Build history of the part. All positions in model axes, mm. Face numbers are marked on the shaded views. A direction names the side the tool comes from. Round coordinates to 2 decimals unless told otherwise and drop trailing zeros. Loops run counter-clockwise (first coordinate to the right, second up) from the corner with the lowest first, then second, coordinate; pieces in that order, holes last. Notation, with made-up numbers: (32.25, 54) - (80.25, 54) arc R27 cw to (80.25, 87) - close; hole circle Ø6 at (-25.5, 69). An arc over 180 degrees is marked (long way). Put each result on its own line as item: value. Start each with the question number.
from build123d import *

# Parameters (mm, degrees)
F1_DEPTH = 50
F2_T     = -4
F3_R     = 15
F3_R_2   = 20
F4_DEPTH = 50.001
F5_R     = 5


with BuildPart() as f1:
    # F0 (on Front) → F1 (new body)
    with BuildSketch(Plane.XZ):
        Polygon((-95, -50), (95, -50), (95, 0), (53.363256, 50), (-95, 50), align=None)
    extrude(amount=-F1_DEPTH)

    # F2
    f2_openings = [f1.faces().sort_by_distance(p)[0] for p in [
        (-95, 25, 0),
        (95, 25, -25),
        (74.181628, 25, 25),
    ]]
    offset(amount=F2_T, openings=f2_openings)

    # F3 (on Front) → F4 (cut, through all)
    with BuildSketch(Plane.XZ):
        with Locations((-70, 25)):
            Circle(F3_R)
        with Locations((65, -20)):
            Circle(F3_R_2)
    extrude(amount=-F4_DEPTH, mode=Mode.SUBTRACT)

    # F5
    f5_edges = [f1.edges().sort_by_distance(p)[0] for p in [
        (-20.818372, 0, 50),
        (-20.818372, 50, 50),
        (0, 0, -50),
        (0, 50, -50),
    ]]
    fillet(f5_edges, radius=F5_R)


solid = f1.part
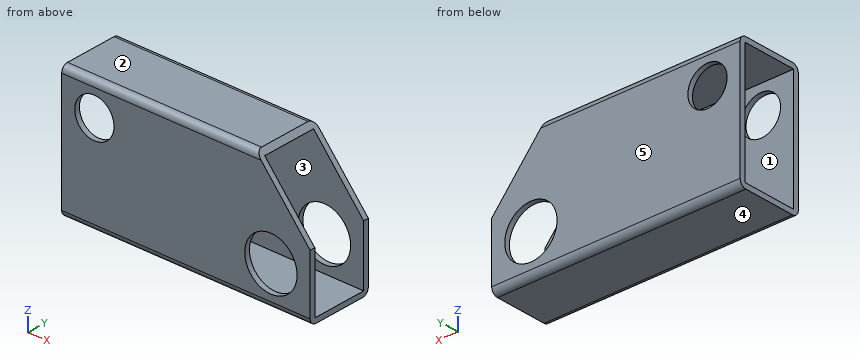
Item 1: Slice it at A-A (y = 8). Give the cut face in (x, z).
Item 2: Slice it at D-D (x = -70). Give the cut face in (y, z).
Item 3: Slice it at B-B (z = -20). Give the cut face in (x, y).
Item 4: Slice it at C-C (x = 27.5). Give the cut face in (y, z).
Item 5: Drill centre lines: probe 1 along Z at (x, y) = (-35, 32.5); probe 2 along Y at (x, z) = (66, 32); probe 3 along Z at (x, y) = (65, 49.15). Where is each one in solid material? Low to high. Write a range as [from, to].
Item 6: Two-plate mould, pull along Z, no slides. Class the marked faces 3, 4 and 5: pulls with the +Z half, pulls with the -Z half, needs draft (parallel to the pull), parting line crosses it, or undercut.
Item 7: Which spindle directions (+Z, -Z, +X, -X, +Y, -Y) get a long thin tool onto all of the face, cutting with end or side? Do the marked faces 1 and 2. Say none if no direction does.
Computed values:
1. outline: (-95, -50) - (95, -50) - (95, -46) - (-95, -46) - close; (-95, 46) - (56.69, 46) - (53.36, 50) - (-95, 50) - close
2. outline: (0, -45) arc R5 ccw to (5, -50) - (45, -50) arc R5 ccw to (50, -45) - (50, 10) - (46, 10) - (46, -46) - (4, -46) - (4, 10) - (0, 10) - close; (0, 40) - (4, 40) - (4, 46) - (46, 46) - (46, 40) - (50, 40) - (50, 45) arc R5 ccw to (45, 50) - (5, 50) arc R5 ccw to (0, 45) - close
3. outline: (-95, 0) - (45, 0) - (45, 4) - (-95, 4) - close; (-95, 46) - (45, 46) - (45, 50) - (-95, 50) - close; (85, 0) - (95, 0) - (95, 4) - (85, 4) - close; (85, 46) - (95, 46) - (95, 50) - (85, 50) - close
4. outline: (0, -45) arc R5 ccw to (5, -50) - (45, -50) arc R5 ccw to (50, -45) - (50, 45) arc R5 ccw to (45, 50) - (5, 50) arc R5 ccw to (0, 45) - close; hole (4, -46) - (46, -46) - (46, 46) - (4, 46) - close
5. probe 1: z = [-50, -46], [46, 50]
5. probe 2: y = [0, 4], [46, 50]
5. probe 3: z = [-47.79, -40], [0, 36.03]
6. face 3: undercut
6. face 4: pulls with the -Z half
6. face 5: needs draft
7. face 1: +X, -X
7. face 2: +Z, +X, -X, +Y, -Y
